Geometry: see drawing. Coordinates: mm, zero at the bounding-box minimum. Round coordinates to 2 decimals unless told otherwise and drop trailing zeros. Write each loop counter-clockwise with the first axis right and the second up, starting at its lowest first coordinate (ties: lowest second). Pieces come first, ordered by that corner, then holes.
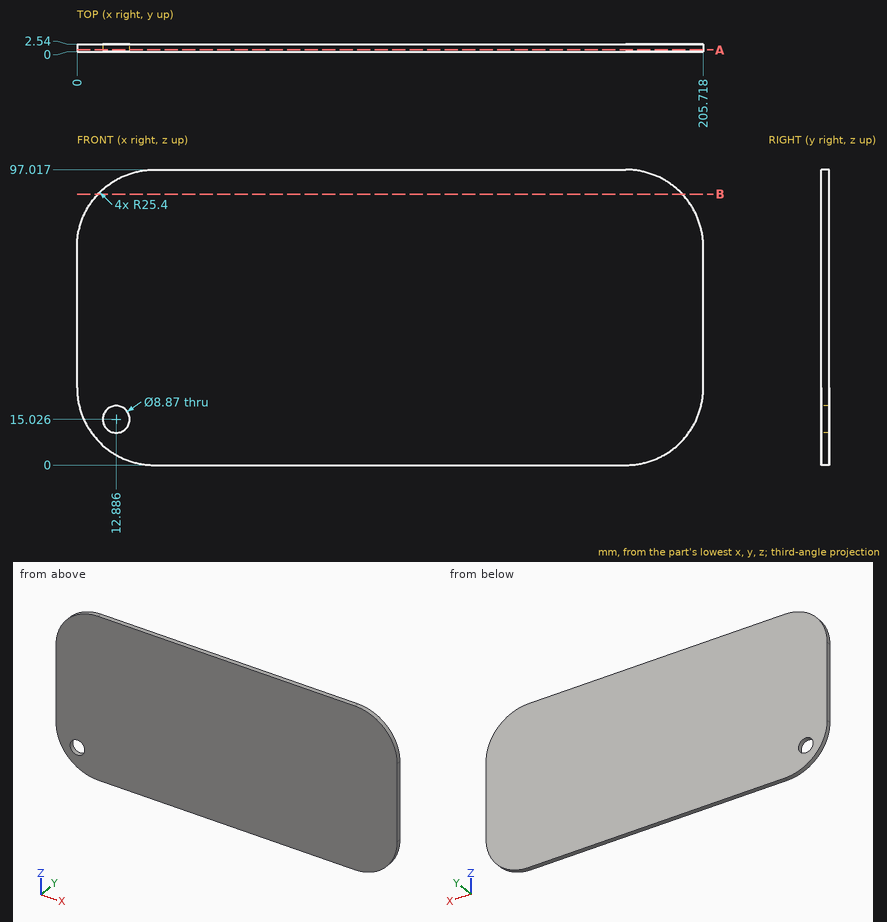
1) Section query B-B on z = 89. Return the cut outline in (x, y).
Taken from the geometry:
outline: (6.88, 0) - (198.84, 0) - (198.84, 2.54) - (6.88, 2.54) - close
2) Contact query for a flat-ended pin moving along its axis: P1, Ø1, axis at y = 2, z = 16.5, coming from the -X side. Output: stop coordinate, or through.
Taken from the geometry:
P1: stops at x = 1.43
3) Section query A-A on y = 0.6. Return the cut outline in (x, z) (1 decimal).
Taken from the geometry:
outline: (0, 25.4) arc R25.4 ccw to (25.4, 0) - (180.3, 0) arc R25.4 ccw to (205.7, 25.4) - (205.7, 71.6) arc R25.4 ccw to (180.3, 97) - (25.4, 97) arc R25.4 ccw to (0, 71.6) - close; hole circle Ø8.9 at (12.9, 15)
4) Material intervals for line 1 (X direction, y = 1.5, z = 15.5) (1 decimal); line 2 (Z direction, x = 10.5, y = 0.7) (1 decimal); line 3 (X direction, y = 2.25, z = 14) (1 decimal), sorted ascending.
Taken from the geometry:
line 1: x = 2 to 8.5, 17.3 to 203.7
line 2: z = 4.8 to 11.3, 18.8 to 92.2
line 3: x = 2.7 to 8.6, 17.2 to 203
